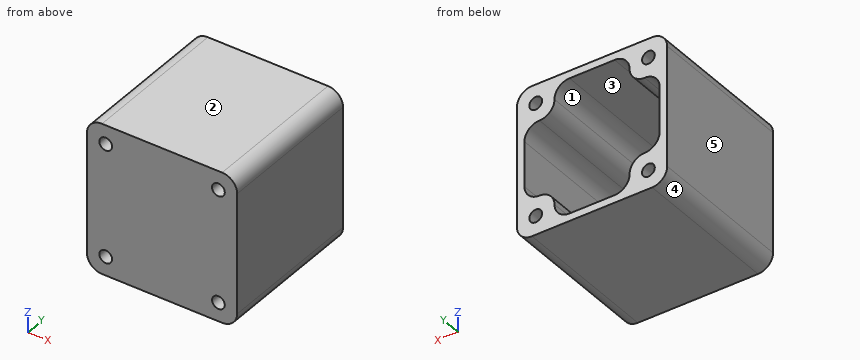
```python
from build123d import *

# Parameters (mm, degrees)
SKETCH1_W           = 40
SKETCH1_H           = 40
SKETCH1_R           = 1.7
BOSS_EXTRUDE1_DEPTH = 40
SKETCH2_W           = 36
SKETCH2_H           = 20
CUT_EXTRUDE1_DEPTH  = 38
CIRPATTERN1_COUNT   = 2
CIRPATTERN1_ANGLE   = 90
FILLET1_R           = 4


with BuildPart() as part:
    # Sketch1 → Boss-Extrude1 (new body)
    with BuildSketch(Plane(origin=(0, 0, 0), x_dir=(1, 0, 0), z_dir=(0, 1, 0))):
        Rectangle(SKETCH1_W, SKETCH1_H)
        with Locations(Location((15, 15, 0), (0, 0, 270))):
            Circle(SKETCH1_R, mode=Mode.SUBTRACT)
        with Locations(Location((-15, 15, 0), (0, 0, 270))):
            Circle(SKETCH1_R, mode=Mode.SUBTRACT)
        with Locations(Location((-15, -15, 0), (0, 0, 270))):
            Circle(SKETCH1_R, mode=Mode.SUBTRACT)
        with Locations(Location((15, -15, 0), (0, 0, 270))):
            Circle(SKETCH1_R, mode=Mode.SUBTRACT)
    extrude(amount=BOSS_EXTRUDE1_DEPTH)

    # Sketch2 → Cut-Extrude1 (cut)
    with BuildSketch(Plane(origin=(0, 40, 0), x_dir=(1, 0, 0), z_dir=(0, 1, 0))):
        Rectangle(SKETCH2_W, SKETCH2_H)
    cut_extrude1 = extrude(amount=-CUT_EXTRUDE1_DEPTH, mode=Mode.SUBTRACT)

    # CirPattern1: Cut-Extrude1 ×2 about axis
    cirpattern1_axis = Axis((0, 0, 0), (0, -1, 0))
    for i in range(1, CIRPATTERN1_COUNT):
        add(cut_extrude1.rotate(cirpattern1_axis, i * CIRPATTERN1_ANGLE / (CIRPATTERN1_COUNT - 1)), mode=Mode.SUBTRACT)

    # Fillet1
    fillet1_edges = [part.edges().sort_by_distance(p)[0] for p in [
        (-18, 21, 10),
        (-10, 21, 10),
        (-10, 21, 18),
        (10, 21, 18),
        (10, 21, 10),
        (18, 21, 10),
        (18, 21, -10),
        (10, 21, -10),
        (10, 21, -18),
        (-10, 21, -18),
        (-18, 21, -10),
        (-10, 21, -10),
        (-20, 20, -20),
        (20, 20, -20),
        (20, 20, 20),
        (-20, 20, 20),
    ]]
    fillet(fillet1_edges, radius=FILLET1_R - 0.0001)  # a hair under: the kernel refuses the full size


solid = part.part
```
Part model, mm, in its own coordinate system. Face numbers are marked on the shaded views. A direction names the side the tool comes from. Give positions to 0.01 mm unless a question says otherwise; leave off trailing zeros. Write each loop counter-clockwise with the first axis right and the second up, starting at its lowest first coordinate (ties: lowest second). Pieces come first, ordered by that corner, then holes. Notation, with made-up numbers: M -1,47 L 29,47 A8 cw 29,61 Z; hole C 61,-26 d11. An arc over 180 degrees is marked long. Use CSV: the item, a comma, the result in double quotes.
Item 1: Which spindle directions (+Z, -Z, +X, -X, +Y, -Y) get a long thin tool onto all of the face, cutting with end or side? Do the marked faces 1 and 2. Say none if no direction does.
Taken from the geometry:
face 1,"+Y"
face 2,"+Z, +X, -X, +Y, -Y"
Item 2: Slice it at D-D on z = 4.5. Write the cut outline in (x, y).
Taken from the geometry:
outline,"M -20,0 L 20,0 L 20,40 L 18,40 L 18,2 L -18,2 L -18,40 L -20,40 Z"
Item 3: Slice it at B-B on z = 15. Write the cut outline in (x, y), plus the area to 3 significant figures.
Taken from the geometry:
outline,"M -20,0 L -16.7,0 L -16.7,40 L -20,40 Z; M -13.3,0 L 13.3,0 L 13.3,40 L 9.87,40 L 9.87,2 L -9.87,2 L -9.87,40 L -13.3,40 Z; M 16.7,0 L 20,0 L 20,40 L 16.7,40 Z"
area,"578 mm²"
Item 4: Pin check, flat tips, straight feed: P1, Ø5, axis at x = 7.5, z = -6.5, coming from the +Y side; P2, Ø2.5, axis at x = -15, z = 15, coming from the -Y side. Stop position of each tip, or through.
Taken from the geometry:
P1,"stops at y = 2"
P2,"passes through"
Item 5: Slice it at C-C on x = 4. Write the cut outline in (y, z).
Taken from the geometry:
outline,"M 0,-20 L 40,-20 L 40,-18 L 2,-18 L 2,18 L 40,18 L 40,20 L 0,20 Z"
Item 6: Drill centre lines: probe 1 along X at (y, z) = (28, -1); probe 2 along X at (y, z) = (29.5, 15). Where is each one in solid material? Low to high.
Taken from the geometry:
probe 1,"x = -20 to -18, 18 to 20"
probe 2,"x = -20 to -16.7, -13.3 to -9.87, 9.87 to 13.3, 16.7 to 20"
Item 7: Pull direction Z, two halves, no side cores. Call the marked faces 3, 4 and 5: +Z half, -Z half, draft (parallel to the pull), parting line (faces both ways), or undercut.
Taken from the geometry:
face 3,"undercut"
face 4,"-Z half"
face 5,"draft"
Item 8: Slice it at A-A on x = -15. Write the cut outline in (y, z), plus the area to 3 significant figures.
Taken from the geometry:
outline,"M 0,-20 L 40,-20 L 40,-16.7 L 0,-16.7 Z; M 0,-13.3 L 40,-13.3 L 40,-9.87 L 2,-9.87 L 2,9.87 L 40,9.87 L 40,13.3 L 0,13.3 Z; M 0,16.7 L 40,16.7 L 40,20 L 0,20 Z"
area,"578 mm²"
